```python
from build123d import *

# Parameters (mm, degrees)
SKETCH1_W               = 300
SKETCH1_H               = 300
BOSS_EXTRUDE1_DEPTH     = 10
BOSS_EXTRUDE4_DEPTH     = 30
CUT_EXTRUDE2_DEPTH      = 215.242852856
CUT_EXTRUDE2_DEPTH_BACK = 215.242852856
SKETCH1_11_R            = 5


with BuildPart() as part:
    # Sketch1 → Boss-Extrude1 (new body)
    with BuildSketch(Plane.XY):
        Rectangle(SKETCH1_W, SKETCH1_H)
    extrude(amount=BOSS_EXTRUDE1_DEPTH)

    # Sketch1<6> → Boss-Extrude4 (add)
    with BuildSketch(Plane.XY):
        Polygon((-120, 150), (-150, 150), (-150, -150), (150, -150), (150, 150), align=None)
        Polygon((120, 0), (120, -120), (0, -120), (-120, -120), (-120, 120), (-55.80388173, 120), (0, 120), (120, 120), align=None, mode=Mode.SUBTRACT)
    extrude(amount=-BOSS_EXTRUDE4_DEPTH)

    # Sketch1<11> → Cut-Extrude2 (cut, two sides: drawn at the far end of the back side and taken through both)
    with BuildSketch(Plane.XY.offset(-CUT_EXTRUDE2_DEPTH_BACK)):
        with Locations((80, 95)):
            Circle(SKETCH1_11_R)
        with Locations((-80, 95)):
            Circle(SKETCH1_11_R)
        with Locations((0, 95)):
            Circle(SKETCH1_11_R)
        with Locations((-80, -95)):
            Circle(SKETCH1_11_R)
        with Locations((80, -95)):
            Circle(SKETCH1_11_R)
        with Locations((0, -95)):
            Circle(SKETCH1_11_R)
    extrude(amount=CUT_EXTRUDE2_DEPTH + CUT_EXTRUDE2_DEPTH_BACK, mode=Mode.SUBTRACT)


solid = part.part
```
Part model, mm, in its own coordinate system. A direction names the side the tool comes from. Give positions to 0.01 mm unless a question says otherwise; leave off trailing zeros. Write each loop counter-clockwise with the first axis right and the second up, starting at its lowest first coordinate (ties: lowest second). Pieces come first, ordered by that corner, then holes. Notation, with made-up numbers: (75, 35) -> (81, 35) arc R16 cw to (81, 43) -> close; hole circle Ø7 at (33, 48). An arc over 180 degrees is marked (long way). Put each result on its own line as item: value. Start each with the question number.
Item 1: Cut at B-B (x = 0). List the corners of the cut face in (y, z).
Item 2: Cut at C-C (z = -12.5). List the corners of the cut face in (x, y), then the cut area to 3 significant figures.
Item 3: Which spindle directions (+Z, -Z, +X, -X, +Y, -Y) get a long thin tool onto all of the face, cutting with end or side? Do faces 1 (the face through (-75.381, 93.085, 4.93)), 2 (the face through (-120, -2, -15)). Say none if no direction does.
Item 4: Pull direction X, two halves, no side cores. Call faces 3 (the face through (-150, 2, -10)), 4 (the face through (-2, 120, -15)), 5 (the face through (-135, 2, -30)), 6 (the face through (150, -2, -10)): pulls with the +X half, pulls with the -X half, needs draft (parallel to the pull), parting line crosses it, or undercut.
Item 5: Cut at A-A (y = -95). List the corners of the cut face in (x, z).
Item 6: Cut at D-D (y = 112). List the corners of the cut face in (x, z).
Item 7: Wall check: L1, parallel to Y at x = -80, z = 5; L2, parallel to X at y = -95, z = 4.25; L3, parallel to Y at x = -104.5, z = -3.5. Give the ranges that are in metal, low to high. Write a range as [from, to].
Item 8: Pin check, flat tips, straight feed: pin 1 Ø8 at (x, y) = (80, 95) entering from -Z; pin 2 Ø16 at (x, y) = (-80, 95) entering from -Z; pin 3 Ø11.5 at (x, y) = (-80, -95) entering from +Z. Stop position of each tip, or through.
Answer list:
1. outline: (-150, -30) -> (-120, -30) -> (-120, 0) -> (-100, 0) -> (-100, 10) -> (-150, 10) -> close; (-90, 0) -> (90, 0) -> (90, 10) -> (-90, 10) -> close; (100, 0) -> (120, 0) -> (120, -30) -> (150, -30) -> (150, 10) -> (100, 10) -> close
2. outline: (-150, -150) -> (150, -150) -> (150, 150) -> (-150, 150) -> close; hole (-120, -120) -> (120, -120) -> (120, 120) -> (-120, 120) -> close
2. area: 32,400 mm2
3. face 1: +Z, -Z
3. face 2: -Z
4. face 3: pulls with the -X half
4. face 4: undercut
4. face 5: needs draft
4. face 6: pulls with the +X half
5. outline: (-150, -30) -> (-120, -30) -> (-120, 0) -> (-85, 0) -> (-85, 10) -> (-150, 10) -> close; (-75, 0) -> (-5, 0) -> (-5, 10) -> (-75, 10) -> close; (5, 0) -> (75, 0) -> (75, 10) -> (5, 10) -> close; (85, 0) -> (120, 0) -> (120, -30) -> (150, -30) -> (150, 10) -> (85, 10) -> close
6. outline: (-150, -30) -> (-120, -30) -> (-120, 0) -> (120, 0) -> (120, -30) -> (150, -30) -> (150, 10) -> (-150, 10) -> close
7. L1: y = [-150, -100], [-90, 90], [100, 150]
7. L2: x = [-150, -85], [-75, -5], [5, 75], [85, 150]
7. L3: y = [-150, -120], [120, 150]
8. pin 1: passes through
8. pin 2: stops at z = 0
8. pin 3: stops at z = 10
